Check sheet for the drawn part. Datum: minimum x, y, z corner. Units: mm. A direction names the side the tool comes from. Round coordinates to 2 decimals unless told otherwise and drop trailing zeros. Order: outer loops, then holes, each group sorted by start corner. A loop starts at its lowest first (then second) coordinate and runs counter-clockwise, first axis right, second up.
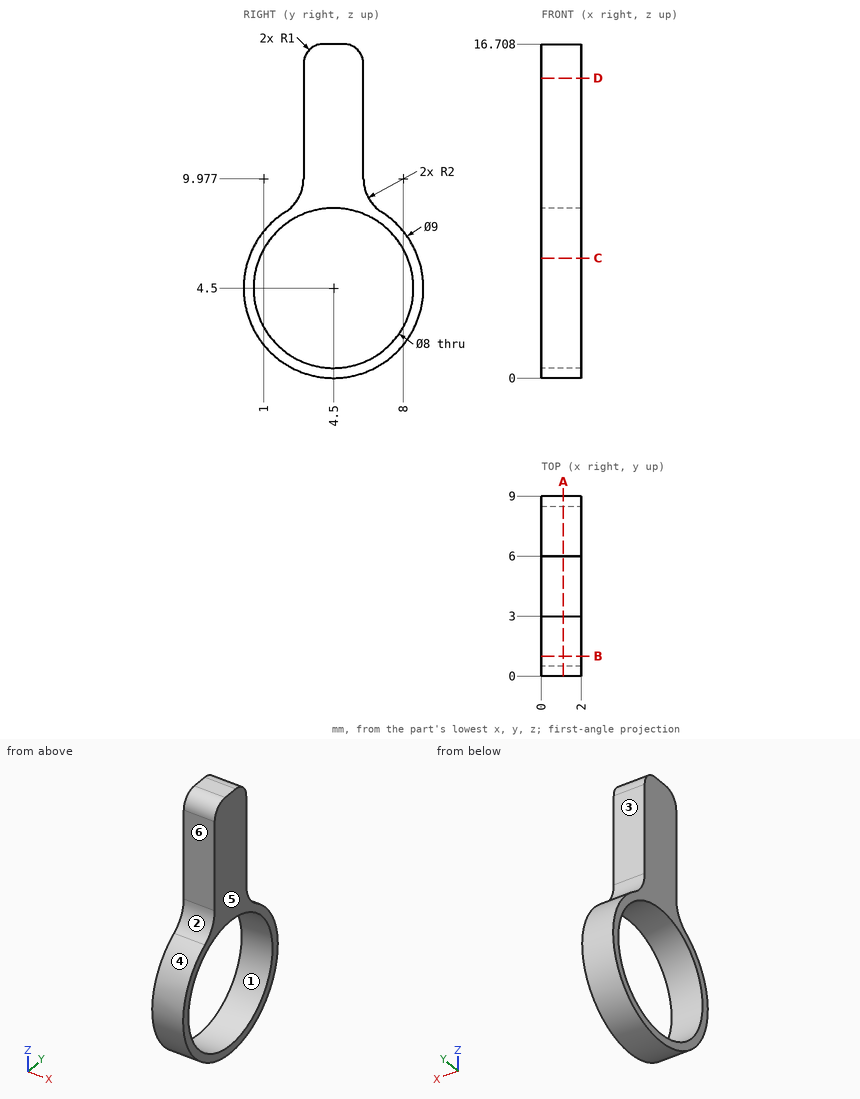
(1) Draft check along Z on the marked faces 1, 2, 3 and 4. Enter one of: released by +Z, released by -Z, zero draft, split by the parting line, or undercut.
Returned:
face 1: undercut
face 2: released by +Z
face 3: zero draft
face 4: split by the parting line
(2) Sectioned sample at B-B, the plane y = 1. Record the cut outline in (x, z).
Returned:
outline: (0, 1.67) - (2, 1.67) - (2, 2.56) - (0, 2.56) - close; (0, 6.44) - (2, 6.44) - (2, 7.33) - (0, 7.33) - close
(3) Sectioned sample at D-D, the plane z = 15. Record the cut outline in (x, y).
Returned:
outline: (0, 3) - (2, 3) - (2, 6) - (0, 6) - close
(4) Sectioned sample at C-C, the plane z = 6. Record the cut outline in (x, y).
Returned:
outline: (0, 0.26) - (2, 0.26) - (2, 0.79) - (0, 0.79) - close; (0, 8.21) - (2, 8.21) - (2, 8.74) - (0, 8.74) - close
(5) Set-up check for the marked faces 5 and 6: record each of +Z, -Z, +X, -X, +Y, -Y from which the full face is reachable in a straight line by a thin tool's end or side.
Returned:
face 5: +Z, -Z, +X, +Y, -Y
face 6: +Z, +X, -X, -Y
(6) Material ranges on line 1 (Y direction, x = 0.95, z = 4.25); line 2 (Y direction, x = 1.95, z = 1) (1 decimal); line 3 (Y direction, x = 0.4, z = 13.25), recorded low to high.
Returned:
line 1: y = 0.01 to 0.51, 8.49 to 8.99
line 2: y = 1.7 to 2.6, 6.4 to 7.3
line 3: y = 3 to 6
(7) Sectioned sample at A-A, the plane x = 1.1. Record the cut outline in (y, z).
Returned:
outline: (2.08, 8.29) arc R4.5 ccw (long way) to (6.92, 8.29) arc R2 cw to (6, 9.98) - (6, 15.71) arc R1 ccw to (5, 16.71) - (4, 16.71) arc R1 ccw to (3, 15.71) - (3, 9.98) arc R2 cw to start; hole circle Ø8 at (4.5, 4.5)
